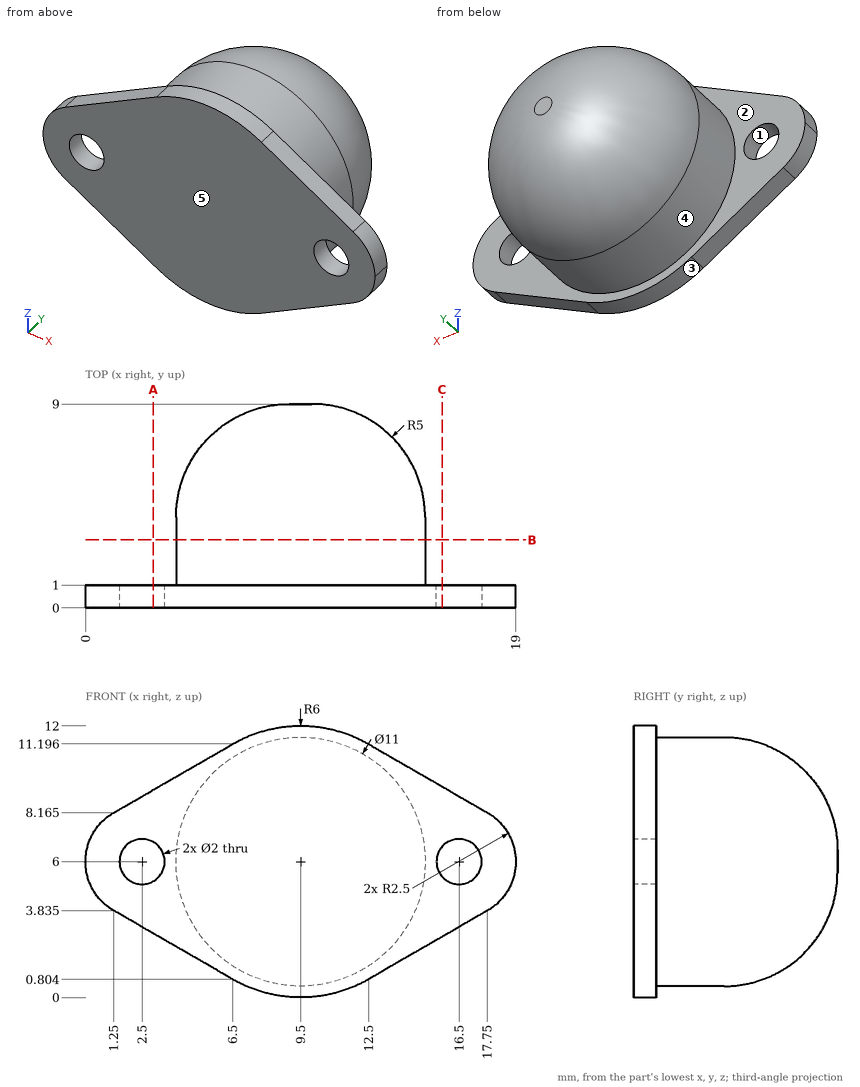
The drawing under review shows one solid part. Ordinate dimensions are in mm from its lowest x, y, z. A direction names the side the tool comes from. Round coordinates to 2 decimals unless told otherwise and drop trailing zeros. Order: outer loops, then holes, each group sorted by start corner. A loop starts at its lowest first (then second) coordinate and runs counter-clockwise, first axis right, second up. Notation, with made-up numbers: (-14, -25) -> (40, -25) arc R26 ccw to (40, -6) -> close; hole circle Ø4 at (-36, 52). An arc over 180 degrees is marked (long way). Use a Markdown table: item, result.
Item 1: Take a section at C-C (x = 15.75). State the section outline as (y, z) points.
Resolved:
| item | result |
|---|---|
| outline | (0, 2.68) -> (1, 2.68) -> (1, 5.34) -> (0, 5.34) -> close; (0, 6.66) -> (1, 6.66) -> (1, 9.32) -> (0, 9.32) -> close |
Item 2: Take a section at B-B (y = 3). State the section outline as (x, z) points.
Resolved:
| item | result |
|---|---|
| outline | circle Ø11 at (9.5, 6) |
Item 3: For line 1 along Z through (x, y) = (16.5, 0.7); line 2 along X through (y, z) = (2, 5.75); line 3 along Y through (x, z) = (16, 4.5), list the stretches that pass through material, from the lowest coordinate up. Write a range as [from, to].
Resolved:
| item | result |
|---|---|
| line 1 | z = [3.11, 5], [7, 8.89] |
| line 2 | x = [4.01, 14.99] |
| line 3 | y = [0, 1] |
Item 4: Draft analysis for pull direction Z (two halves, no side actions). For the marked faces 1, 2 and 3, state which applies: +Z half, -Z half, draft (parallel to the pull), parting line (faces both ways), or undercut.
Resolved:
| item | result |
|---|---|
| face 1 | undercut |
| face 2 | draft |
| face 3 | -Z half |
Item 5: For pin 1 (1.5 mm diameter, centred on x = 16.5, z = 1.5, fed in from -Y); pin 2 (6 mm diameter, centred on x = 2.5, z = 8, fed in from +Y), all flat-tipped, find the tip position at first contact; note any pin that passes through.
Resolved:
| item | result |
|---|---|
| pin 1 | passes through |
| pin 2 | stops at y = 7.27 |
Item 6: Take a section at A-A (x = 3). State the section outline as (y, z) points.
Resolved:
| item | result |
|---|---|
| outline | (0, 2.82) -> (1, 2.82) -> (1, 5.13) -> (0, 5.13) -> close; (0, 6.87) -> (1, 6.87) -> (1, 9.18) -> (0, 9.18) -> close |
Item 7: Machinability: for the marked faces 4 and 5, which of the approach directions +Z, -Z, +X, -X, +Y, -Y give a long, thin tool a straight path to every point of the face, cutting with its end or side? Answer none if there is none.
Resolved:
| item | result |
|---|---|
| face 4 | +Y |
| face 5 | +Z, -Z, +X, -X, -Y |
